The listing builds one solid part. Answer for the finished solid, in the listing's coordinates (mm). A direction names the side the tool comes from. Round coordinates to 2 decimals unless told otherwise and drop trailing zeros. Order: outer loops, then holes, each group sorted by start corner. A loop starts at its lowest first (then second) coordinate and runs counter-clockwise, first axis right, second up. Notation, with made-up numbers: (79.25, -13.5) - (105.25, -13.5) arc R11 ccw to (105.25, 7.5) - close; hole circle Ø8 at (-35, 72). An arc over 180 degrees is marked (long way). Use CSV: the item, a comma, the result in double quotes. Start each with the question number.
Item 1: Find section D-D, the plane y = 30. Give the vertices of the cut face in (x, z).
Item 2: Find section C-C, the plane y = -27. Give the vertices of the cut face in (x, z), plus the area to 3 significant figures.
Item 3: Straight lines are drawn through the part: line 1 along Z through (x, y) = (22, 38); line 2 along X through (y, z) = (19.5, -23); line 3 along X through (y, z) = (-16, -33). For each, find the intervals that lie inside material, in ascending order. Write a range as [from, to].
Item 4: Find section A-A, the plane x = 22.5. Give the vertices of the cut face in (y, z).
Item 5: Find section B-B, the plane z = -22.5. Count the separate pieces of the cut face and the enclosed holes in it, plus the area to 3 significant figures.
Item 6: Determine the mould class of faces 1 (the flat face through (-106, -11, -23)), 2 (the flat face through (22, 0, -3)), 3 (the flat face through (-100, -15, -23)) for opening direction X: +X half, -X half, draft (parallel to the pull), parting line (faces both ways), or undercut.
Item 7: Flat-ended cylindrical pins translate along their axes: P1, Ø1.5, axis at x = 18, y = 31.5, coming from the -Z side; P2, Ø11.5, axis at y = -28.5, z = -27.5, coming from the +X side; P3, Ø2, axis at x = -40, z = -29.5, coming from the +Y side. Find the tip coordinate at first contact, or state that the pin passes through.
Item 8: For faces 4 (the flat face through (-59, 0, -22)), 5 (the flat face through (-13, -38, -22)), 6 (the cylindrical face through (32.31, 17.75, -7.11)), determine the directions among +Z, -Z, +X, -X, +Y, -Y from which every point of the face is accessible in a straight line to the end or side of a thin tool.
Autodesk Inventor part; units mm, degrees
ref_plane "YZ Plane" through (0, 0, 0) normal (1, 0, 0) x (0, 1, 0)
ref_plane "XZ Plane" through (0, 0, 0) normal (0, 1, 0) x (-1, 0, 0)
ref_plane "XY Plane" through (0, 0, 0) normal (0, 0, 1) x (1, 0, 0)
ref_plane "Work Plane3" through (0, 6, 0) normal (0, 1, 0) x (1, 0, 0)
sketch "Sketch2" plane through (0, 6, 0) normal (0, 1, 0) x (1, 0, 0)
  line L0 (0, 0) -> (0, 22.5)
  line L1 (0, 45) -> (0, 0)
  line L2 (0, 22.5) -> (22.5, 22.5)
  circle A0 centre (22.5, 22.5) radius 22.5
  dimension "d5" = 22.5
  dimension "d6" = 22.5
  dimension "d7" = 45
extrude "Extrusion2" add sketch "Sketch2" along normal blind 33.5
ref_plane "Work Plane2" through (0, 0, 0) normal (0, -1, 0) x (1, 0, 0)
sketch "Sketch3" plane through (0, 0, 0) normal (0, -1, 0) x (1, 0, 0)
  line L0 (0, -45) -> (0, 0)
  line L1 (0, 0) -> (0, -22.5)
  circle A0 centre (22.5, -22.5) radius 18.25
  dimension "d12" = 36.5
extrude "Extrusion3" cut sketch "Sketch3" against normal blind 65
sketch "Sketch4" plane through (22.5, 39.5, -22.5) normal (0, 1, 0) x (1, 0, 0)
  circle A0 centre (0, 0) radius 6.75
  point P0 (-22.5, -22.5)
  dimension "d15" = 13.5
extrude "Extrusion4" cut sketch "Sketch4" against normal blind 4.5
ref_plane "Work Plane1" through (0, 0, 0) normal (0, -1, 0) x (1, 0, 0)
sketch "Sketch5" plane through (0, 0, 0) normal (0, -1, 0) x (1, 0, 0)
  line L0 (0, -45) -> (0, 0)
  line L1 (0, 0) -> (22.5, 0)
  line L2 (0, 0) -> (45, 0)
sketch "Sketch6" plane through (22.5, 39.5, -22.5) normal (0, 1, 0) x (1, 0, 0)
  point P0 (-22.5, -22.5)
sketch "Sketch7" plane through (22.5, 39.5, -22.5) normal (0, 1, 0) x (1, 0, 0)
  circle A0 centre (0, 0) radius 18.25
  circle A1 centre (0, 0) radius 18.25
  point P0 (-22.5, -22.5)
extrude "Extrusion5" add sketch "Sketch7" against normal blind 3.5
sketch "Sketch8" plane through (22.5, 39.5, -22.5) normal (0, 1, 0) x (1, 0, 0)
  circle A0 centre (0, 0) radius 6.75
  point P0 (-22.5, -22.5)
  dimension "d20" = 13.5
extrude "Extrusion6" cut sketch "Sketch8" against normal blind 3.5
sketch "Sketch9" plane through (22.5, 6, -22.5) normal (0, -1, 0) x (1, 0, 0)
  point P0 (-22.5, 22.5)
sketch "Sketch10" plane through (22.5, 39.5, -22.5) normal (0, 1, 0) x (1, 0, 0)
  point P0 (-22.5, -22.5)
sketch "Sketch11" plane through (22.5, 6, -22.5) normal (0, -1, 0) x (1, 0, 0)
  circle A0 centre (0, 0) radius 22.5
  line L0 (0, 29) -> (32.5, 29)
  line L1 (32.5, 29) -> (32.5, -29)
  line L2 (32.5, -29) -> (-32.5, -29)
  line L3 (0, 29) -> (-32.5, 29)
  line L4 (-32.5, -29) -> (-128.5, -29)
  line L5 (-128.5, -29) -> (-128.5, 29)
  line L6 (-128.5, 29) -> (-32.5, 29)
  point P0 (-22.5, 22.5)
  dimension "d25" = 58
  dimension "d26" = 65
  dimension "d27" = 32.5
  dimension "d28" = 96
sketch "Sketch12" plane through (22.5, 6, -22.5) normal (0, -1, 0) x (1, 0, 0)
  point P0 (-22.5, 22.5)
extrude "Extrusion7" add sketch "Sketch11" along normal blind 6
sketch "Sketch13" plane through (22.5, 6, -22.5) normal (0, -1, 0) x (1, 0, 0)
  circle A0 centre (0, 0) radius 6.75
  circle A1 centre (0, 0) radius 22.5
  point P0 (-22.5, 22.5)
extrude "Extrusion8" add sketch "Sketch13" along normal blind 6 contours A0 | A1
sketch "Sketch14" plane through (22.5, 0, -22.5) normal (0, -1, 0) x (1, 0, 0)
  circle A0 centre (0, 0) radius 18.25
  point P0 (-22.5, 22.5)
extrude "Extrusion9" cut sketch "Sketch14" against normal blind 6
sketch "Sketch15" plane through (-106, 6, -51.5) normal (-1, 0, 0) x (0, 0, 1)
  line L0 (58, -6) -> (0, -6)
  line L1 (29, -42) -> (38, -42)
  line L2 (29, -42) -> (20, -42)
  line L3 (20, -42) -> (0, -6)
  line L4 (38, -42) -> (58, -6)
  circle A0 centre (29, -33) radius 5
  point P0 (51.5, -6)
  dimension "d38" = 18
  dimension "d41" = 10
extrude "Extrusion10" add sketch "Sketch15" against normal blind 6
sketch "Sketch17" plane through (-106, -36, -31.5) normal (0, -1, 0) x (1, 0, 0)
  point P0 (106, 31.5)
sketch "Sketch18" plane through (-106, -36, -31.5) normal (0, -1, 0) x (1, 0, 0)
  line L0 (6, 18) -> (6, 0)
  line L1 (6, 18) -> (0, 18)
  line L2 (0, 38) -> (0, -20)
  line L3 (0, 0) -> (6, 0)
  line L4 (6, 0) -> (6, 18)
  line L5 (0, 18) -> (0, 0)
  point P0 (106, 31.5)
extrude "Extrusion12" add sketch "Sketch18" along normal blind 2
sketch "Sketch19" plane through (-106, 6, -51.5) normal (-1, 0, 0) x (0, 0, 1)
  line L0 (38, -42) -> (38, -44)
  line L1 (38, -44) -> (40, -44)
  line L2 (58, -44) -> (0, -44)
  line L3 (38, -42) -> (58, -6)
  line L4 (40, -44) -> (58, -6)
  line L5 (58, -6) -> (38, -42)
  line L6 (38, -42) -> (38, -44)
  line L7 (40, -44) -> (38, -44)
  point P0 (51.5, -6)
  dimension "d53" = 2
extrude "Extrusion13" add sketch "Sketch19" against normal blind 6
sketch "Sketch20" plane through (-106, 6, -51.5) normal (-1, 0, 0) x (0, 0, 1)
  line L0 (20, -42) -> (20, -44)
  line L1 (20, -44) -> (18, -44)
  line L2 (58, -44) -> (0, -44)
  line L3 (0, -6) -> (20, -42)
  line L4 (18, -44) -> (0, -6)
  line L5 (0, -6) -> (20, -42)
  line L6 (20, -42) -> (20, -44)
  line L7 (18, -44) -> (20, -44)
  point P0 (51.5, -6)
  dimension "d56" = 2
extrude "Extrusion14" add sketch "Sketch20" against normal blind 6
sketch "Sketch24" plane through (55, 6, -51.5) normal (0, 0, -1) x (-1, 0, 0)
  line L0 (155, -6) -> (0, -6)
  point P0 (55, -6)
  point P1 (61, -6)
sketch "Sketch25" plane through (22.5, 0, -22.5) normal (0, -1, 0) x (1, 0, 0)
  line L0 (-32.5, -29) -> (-38.5, -29)
  line L1 (-38.5, -29) -> (-38.5, 29)
  line L2 (32.5, 29) -> (-122.5, 29)
  line L3 (-38.5, 29) -> (-32.5, 29)
  line L4 (-32.5, 29) -> (-32.5, -29)
  point P0 (-22.5, 22.5)
  dimension "d71" = 6
  dimension "d72" = 6
extrude "Extrusion18" add sketch "Sketch25" along normal blind 38
sketch "Sketch26" plane through (-10, 0, 6.5) normal (1, 0, 0) x (0, 0, -1)
  line L0 (0, 0) -> (58, 0)
  circle A0 centre (29, -27) radius 5
  point P0 (6.5, 0)
  dimension "d76" = 10
sketch "Sketch27" plane through (-10, 0, 6.5) normal (1, 0, 0) x (0, 0, -1)
  point P0 (6.5, 0)
extrude "Extrusion19" cut sketch "Sketch26" against normal blind 6
sketch "Sketch28" plane through (-10, 0, 6.5) normal (1, 0, 0) x (0, 0, -1)
  circle A0 centre (29, -27) radius 5
  line L0 (58, 0) -> (58, -38)
  line L1 (40, -38) -> (58, 0)
  line L2 (58, 0) -> (58, -38)
  line L3 (58, -38) -> (40, -38)
  point P0 (6.5, 0)
extrude "Extrusion20" cut sketch "Sketch28" against normal blind 6 contours L0 L3 L1
sketch "Sketch29" plane through (-10, -38, 6.5) normal (1, 0, 0) x (0, 0, -1)
  circle A0 centre (29, 11) radius 5
  line L0 (0, 38) -> (18, 0)
  line L1 (18, 0) -> (0, 38)
  line L2 (0, 38) -> (0, 0)
  line L3 (0, 38) -> (0, 0)
  line L4 (0, 0) -> (18, 0)
  point P0 (6.5, 38)
extrude "Extrusion21" cut sketch "Sketch29" against normal blind 6 contours L0 L4 L2
sketch "Sketch30" plane through (55, 6, -51.5) normal (0, 0, -1) x (-1, 0, 0)
  point P0 (55, -6)
properties part number "angleadjuster"
Worked out:
1,outline,"circle Ø45 at (22.5, -22.5); hole circle Ø36.5 at (22.5, -22.5)"
2,outline,"(-106, -38.71) - (-100, -38.71) - (-100, -27.5) - (-106, -27.5) - close; (-106, -17.5) - (-100, -17.5) - (-100, -6.29) - (-106, -6.29) - close; (-16, -38.71) - (-10, -38.71) - (-10, -27.5) - (-16, -27.5) - close; (-16, -17.5) - (-10, -17.5) - (-10, -6.29) - (-16, -6.29) - close"
2,area,"269 mm²"
3,line 1,"z = [-44.99, -29.23], [-15.77, -0.01]"
3,line 2,"x = [0.01, 4.26], [40.74, 44.99]"
3,line 3,"x = [-106, -100], [-16, -10]"
4,outline,"(0, -51.5) - (6, -51.5) - (6, -45) - (39.5, -45) - (39.5, -29.25) - (36, -29.25) - (36, -40.75) - (0, -40.75) - close; (0, -4.25) - (36, -4.25) - (36, -15.75) - (39.5, -15.75) - (39.5, 0) - (6, 0) - (6, 6.5) - (0, 6.5) - close"
5,separate pieces,"4"
5,enclosed holes,"0"
5,area,"1,450 mm²"
6,face 1,"-X half"
6,face 2,"draft"
6,face 3,"undercut"
7,P1,"stops at z = -44.69"
7,P2,"stops at x = -10"
7,P3,"stops at y = 6"
8,face 4,"+Z, -Z, -Y"
8,face 5,"+Z, -Z, +X, -X, -Y"
8,face 6,"-Y"
